```python
from build123d import *

# Parameters (mm, degrees)
SKETCH1_R               = 2
BOSS_EXTRUDE1_DEPTH     = 150
BOSS_EXTRUDE2_START     = 28
BOSS_EXTRUDE2_OUTLINE_R = 8
BOSS_EXTRUDE2_DEPTH     = 8


# Read off the part's stored shape, not the designer's step: Boss-Extrude2
with BuildPart() as part:
    # Sketch1 → Boss-Extrude1 (new body)
    with BuildSketch(Plane(origin=(0, 0, 0), x_dir=(0, 0, -1), z_dir=(1, 0, 0))):
        Circle(SKETCH1_R)
    extrude(amount=BOSS_EXTRUDE1_DEPTH)

    # Boss-Extrude2 outline → Boss-Extrude2 (add)
    with BuildSketch(Plane.YZ.offset(BOSS_EXTRUDE2_START)):
        with Locations((-0.186353815, 0)):
            Circle(BOSS_EXTRUDE2_OUTLINE_R)
    extrude(amount=BOSS_EXTRUDE2_DEPTH)


solid = part.part
```
For this review, take the finished solid that the model builds, in its own axes (mm). A direction names the side the tool comes from. Coordinates: 2 decimals unless noted, no trailing zeros. Order: outer loops, then holes, each group sorted by start corner. A loop starts at its lowest first (then second) coordinate and runs counter-clockwise, first axis right, second up. Notation, with made-up numbers: (-29.75, 16.25) -> (-10.75, 16.25) arc R18 cw to (-10.75, 50.25) -> close; hole circle Ø11 at (82.5, -20). An arc over 180 degrees is marked (long way). Answer as CSV lines item,"result".
Q1. We need section D-D (z = 6.5). State the section outline as (x, y) points, plus the area to 3 significant figures.
Model answer:
outline,"(28, -4.85) -> (36, -4.85) -> (36, 4.48) -> (28, 4.48) -> close"
area,"74.6 mm2"
Q2. We need section A-A (z = 0). State the section outline as (x, y) points, plus the area to 3 significant figures.
Model answer:
outline,"(0, -2) -> (28, -2) -> (28, -8.19) -> (36, -8.19) -> (36, -2) -> (150, -2) -> (150, 2) -> (36, 2) -> (36, 7.81) -> (28, 7.81) -> (28, 2) -> (0, 2) -> close"
area,"696 mm2"
Q3. We need section C-C (x = 71). State the section outline as (y, z) points, plus the area to 3 significant figures.
Model answer:
outline,"circle Ø4 at (0, 0)"
area,"12.6 mm2"
Q4. Clearance check with flat-ended pins moving along their axes: pin 1 Ø8 at (y, z) = (0, -3.5) entering from -X; pin 2 Ø1 at (y, z) = (2.5, -6) entering from -X; pin 3 Ø8 at (x, z) = (103, -3) entering from +Y; pin 4 Ø3 at (x, y) = (42, -2.5) entering from -Z. State where each tip first meets the part, or that it passes through.
Model answer:
pin 1,"stops at x = 0"
pin 2,"stops at x = 28"
pin 3,"stops at y = 2"
pin 4,"stops at z = -1.73"
Q5. For faces 1 (the face through (14, -2, 0)), 2 (the face through (92, -2, 0)), 3 (the face through (0, 0, 0)), list the 3-axis set-ups (+Z, -Z, +X, -X, +Y, -Y) from which the entire face can be reached by the end or side of a thin tool; tool diameter is ignored.
Model answer:
face 1,"-X"
face 2,"+X"
face 3,"+Z, -Z, -X, +Y, -Y"
Q6. Wall thickness on line 1 along X through (y, z) = (7.25, 1.25); line 2 along Z through (x, y) = (14, 0); line 3 along Z through (x, y) = (116, 0.75): over which ranges is each line inside the solid? List them lowest first. Write a range as [from, to].
Model answer:
line 1,"x = [28, 36]"
line 2,"z = [-2, 2]"
line 3,"z = [-1.85, 1.85]"
Q7. We need section B-B (y = 0). State the section outline as (x, z) points, plus the area to 3 significant figures.
Model answer:
outline,"(0, -2) -> (28, -2) -> (28, -8) -> (36, -8) -> (36, -2) -> (150, -2) -> (150, 2) -> (36, 2) -> (36, 8) -> (28, 8) -> (28, 2) -> (0, 2) -> close"
area,"696 mm2"
